Autodesk Inventor part; units mm, degrees
ref_plane "Plano de trabajo1" through (0, 14.2, 0) normal (0, 1, 0) x (1, 0, 0)
ref_plane "YZ Plane" through (0, 0, 0) normal (1, 0, 0) x (0, 1, 0)
ref_plane "XZ Plane" through (0, 0, 0) normal (0, 1, 0) x (-1, 0, 0)
sketch "Boceto1" plane through (0, 0, 0) normal (0, 1, 0) x (-1, 0, 0)
  circle A0 centre (0, 0) radius 26
  dimension "d0" = 52
extrude "Extrusión1" add sketch "Boceto1" along normal blind 4
sketch "Boceto2" plane through (0, 4, 0) normal (0, 1, 0) x (1, 0, 0)
  circle A0 centre (0, 0) radius 21.775
  dimension "d3" = 43.55
extrude "Extrusión2" add sketch "Boceto2" along normal blind 13.8
sketch "Boceto3" plane through (0, 17.8, 0) normal (0, 1, 0) x (1, 0, 0)
  circle A0 centre (0, 0) radius 13.875
  dimension "d6" = 27.75
extrude "Extrusión3" cut sketch "Boceto3" against normal blind 7.85
sketch "Boceto4" plane through (0, 9.95, 0) normal (0, 1, 0) x (1, 0, 0)
  circle A0 centre (0, 0) radius 4.8
  dimension "d9" = 9.6
extrude "Extrusión4" cut sketch "Boceto4" against normal blind 12
sketch "Boceto5" plane through (0, 0, 0) normal (0, -1, 0) x (1, 0, 0)
  circle A0 centre (0, 0) radius 21.2
  dimension "d12" = 42.4
extrude "Extrusión5" cut sketch "Boceto5" against normal blind 3
thread "Rosca1"
ref_plane "Plano de trabajo1" through (0, 14.2, 0) normal (0, 1, 0) x (1, 0, 0)
sketch "Boceto6" plane through (0, 14.2, 0) normal (0, 1, 0) x (1, 0, 0)
  circle A0 centre (0, 0) radius 21.775
  circle A1 centre (0, 0) radius 18.925
  dimension "d18" = 37.85
extrude "Extrusión6" cut sketch "Boceto6" against normal blind 5
properties part number "Pieza_sonar"
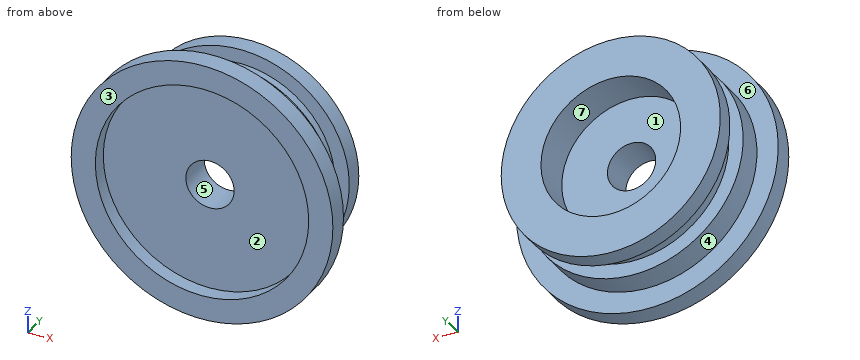
Build history of the part. All positions in model axes, mm. Face numbers are marked on the shaded views. A direction names the side the tool comes from. Give positions to 0.01 mm unless a question says otherwise; leave off trailing zeros. Loops run counter-clockwise (first coordinate to the right, second up) from the corner with the lowest first, then second, coordinate; pieces in that order, holes last.
1) Two-plate mould, pull along X, no slides. Class the marked faces 4, 5, 6 and 7: released by +X, released by -X, zero draft, split by the parting line, or undercut.
Values follow:
face 4: split by the parting line
face 5: undercut
face 6: zero draft
face 7: undercut
2) Probe line 1 along Y through (x, z) = (1.5, 21); line 2 along X through (y, z) = (6, 0) (3 decimals); line 3 along Z through (x, y) = (0, 12.5) (3 decimals). List the from-to ranges inside material, lowest first.
Values follow:
line 1: y = 3 to 9.2, 14.2 to 17.8
line 2: x = -21.775 to -4.8, 4.8 to 21.775
line 3: z = -18.925 to -13.875, 13.875 to 18.925
3) 3-axis set-ups, long thin cutter, end or side, ignore diameter. For the marked faces 1, 2 and 3: which of +Z, -Z, +X, -X, +Y, -Y reach the whole face in a straight line?
Values follow:
face 1: +Y
face 2: -Y
face 3: +Z, -Z, +X, -X, -Y
4) Band-saw the part on A-A on z = 0. List the corners of the cut face in (x, y) (3 decimals).
Values follow:
outline: (-26, 0) - (-21.2, 0) - (-21.2, 3) - (-4.8, 3) - (-4.8, 9.95) - (-13.875, 9.95) - (-13.875, 17.8) - (-21.775, 17.8) - (-21.775, 14.2) - (-18.925, 14.2) - (-18.925, 9.2) - (-21.775, 9.2) - (-21.775, 4) - (-26, 4) - close; (4.8, 3) - (21.2, 3) - (21.2, 0) - (26, 0) - (26, 4) - (21.775, 4) - (21.775, 9.2) - (18.925, 9.2) - (18.925, 14.2) - (21.775, 14.2) - (21.775, 17.8) - (13.875, 17.8) - (13.875, 9.95) - (4.8, 9.95) - close
5) Band-saw the part on D-D on z = 8. List the corners of the cut face in (x, y).
Values follow:
outline: (-24.74, 0) - (-19.63, 0) - (-19.63, 3) - (19.63, 3) - (19.63, 0) - (24.74, 0) - (24.74, 4) - (20.25, 4) - (20.25, 9.2) - (17.15, 9.2) - (17.15, 14.2) - (20.25, 14.2) - (20.25, 17.8) - (11.34, 17.8) - (11.34, 9.95) - (-11.34, 9.95) - (-11.34, 17.8) - (-20.25, 17.8) - (-20.25, 14.2) - (-17.15, 14.2) - (-17.15, 9.2) - (-20.25, 9.2) - (-20.25, 4) - (-24.74, 4) - close
6) Drop flat-ended pins along their axis: P1, Ø8, axis at x = -11, y = 3.5, coming from the +Z side; P2, Ø10, axis at x = -6.5, y = 6.5, coming from the -Z side; P3, Ø1, axis at x = -10, y = 5.5, coming from the +Z side. Give the stop position or say it passes through.
Values follow:
P1: stops at z = 25.04
P2: stops at z = -25.91
P3: stops at z = 19.59
7) Band-saw the part on C-C on y = 8.5. List the corners of the cut face in (x, z) (3 decimals).
Values follow:
outline: circle Ø43.55 at (0, 0); hole circle Ø9.6 at (0, 0)
8) Band-saw the part on B-B on x = 0. List the corners of the cut face in (y, z) (3 decimals).
Values follow:
outline: (0, -26) - (4, -26) - (4, -21.775) - (9.2, -21.775) - (9.2, -18.925) - (14.2, -18.925) - (14.2, -21.775) - (17.8, -21.775) - (17.8, -13.875) - (9.95, -13.875) - (9.95, -4.8) - (3, -4.8) - (3, -21.2) - (0, -21.2) - close; (0, 21.2) - (3, 21.2) - (3, 4.8) - (9.95, 4.8) - (9.95, 13.875) - (17.8, 13.875) - (17.8, 21.775) - (14.2, 21.775) - (14.2, 18.925) - (9.2, 18.925) - (9.2, 21.775) - (4, 21.775) - (4, 26) - (0, 26) - close
